For this review, use the dimensioned drawing (mm, ordinates from the lowest corner) and the shaded views. Round coordinates to 2 decimals unless told otherwise and drop trailing zeros. Loops run counter-clockwise (first coordinate to the right, second up) from the corner with the lowest first, then second, coordinate; pieces in that order, holes last. Notation, with made-up numbers: M 24,56 L 76,56 A5 cw 76,65 Z; hole C 81.25,-34 d4. An arc over 180 degrees is marked long. Use a Markdown table: item, result. Add a question column.
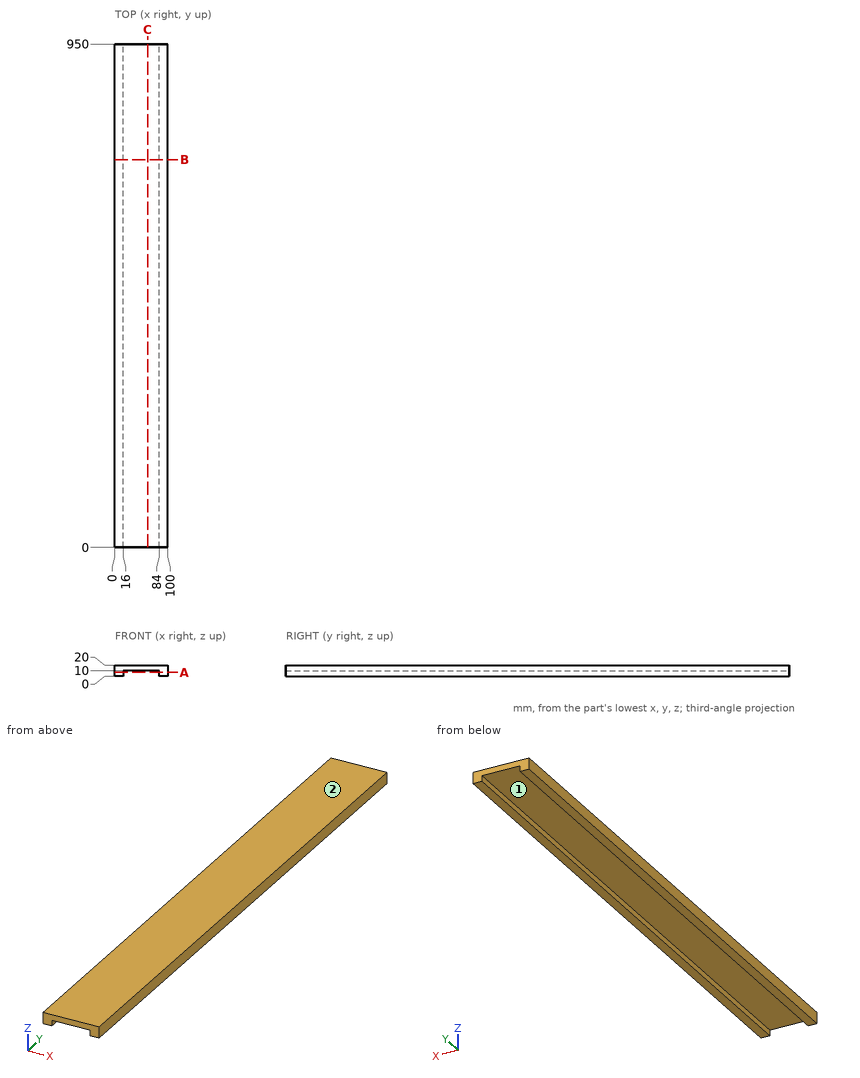
(1) Insertion check: pin 1 Ø5 at (x, y) = (38.5, 124) entering from -Z; pin 2 Ø1 at (x, z) = (43.5, 9) entering from +Y. Each pin has a flat end and moves straight along its axis. Give the tip position at first contact, or say it passes through.
(2) Draft analysis for pull direction X (two halves, no side actions). For the marked faces 1 and 2, state which applies: released by +X, released by -X, zero draft, split by the parting line, or undercut.
(3) To check wall thickness, follow probe 1 along X at (y, z) = (346.5, 6.25); probe 2 along Z at (x, y) = (30, 420). State the ranges of each line that lie inside material, in increasing order.
(4) Consider section B-B, the plane y = 732. Give the boundary of the cut face in (x, z).
(5) Consider section C-C, the plane x = 62. Give the boundary of the cut face in (y, z), then the cut area to 3 significant figures.
(6) Consider section A-A, the plane z = 6.75. Give the boundary of the cut face in (x, y).
Found:
| question | item | result |
|---|---|---|
| 1 | pin 1 | stops at z = 10 |
| 1 | pin 2 | passes through |
| 2 | face 1 | undercut |
| 2 | face 2 | zero draft |
| 3 | probe 1 | x = 0 to 16, 84 to 100 |
| 3 | probe 2 | z = 10 to 20 |
| 4 | outline | M 0,0 L 16,0 L 16,10 L 84,10 L 84,0 L 100,0 L 100,20 L 0,20 Z |
| 5 | outline | M 0,10 L 950,10 L 950,20 L 0,20 Z |
| 5 | area | 9,500 mm^2 |
| 6 | outline | M 0,0 L 16,0 L 16,950 L 0,950 Z; M 84,0 L 100,0 L 100,950 L 84,950 Z |
